from build123d import *

# Parameters (mm, degrees)
SKETCH2_R           = 2
BOSS_EXTRUDE1_DEPTH = 2.5
FILLET1_R           = 4
FILLET2_R           = 2


with BuildPart() as part:
    # Sketch2 → Boss-Extrude1 (new body)
    with BuildSketch(Plane.XY.offset(38.1)):
        Polygon((-27.5, 0), (27.5, 0), (27.5, 59.920564885), (-7.5, 59.920564885), (-7.5, 47.920564885), (15.5, 47.920564885), (15.5, 25.623759218), (1.876240782, 12), (-15.5, 12), (-15.5, 24), (-27.5, 24), (-27.5, 12), align=None)
        with Locations((-3.5, 56.920564885)):
            Circle(SKETCH2_R, mode=Mode.SUBTRACT)
        with Locations((-3.5, 50.920564885)):
            Circle(SKETCH2_R, mode=Mode.SUBTRACT)
        with Locations((4.5, 50.920564885)):
            Circle(SKETCH2_R, mode=Mode.SUBTRACT)
        with Locations((12.5, 50.920564885)):
            Circle(SKETCH2_R, mode=Mode.SUBTRACT)
        with Locations((4.5, 56.920564885)):
            Circle(SKETCH2_R, mode=Mode.SUBTRACT)
        with Locations((12.5, 56.920564885)):
            Circle(SKETCH2_R, mode=Mode.SUBTRACT)
        with Locations((20.5, 56.920564885)):
            Circle(SKETCH2_R, mode=Mode.SUBTRACT)
        Polygon((23.5, 4), (23.5, 47.920564885), (19.5, 47.920564885), (19.5, 23.966904969), (3.533095031, 8), (-19.190748402, 8), (-19.190748402, 20), (-23.5, 20), (-23.5, 8), (-23.5, 4), align=None, mode=Mode.SUBTRACT)
    extrude(amount=BOSS_EXTRUDE1_DEPTH)

    # Fillet1
    fillet1_edges = [part.edges().sort_by_distance(p)[0] for p in [
        (15.5, 25.623759218, 39.35),
        (15.5, 47.920564885, 39.35),
        (27.5, 0, 39.35),
        (-27.5, 0, 39.35),
        (-27.5, 24, 39.35),
        (-15.5, 24, 39.35),
        (-15.5, 12, 39.35),
        (1.876240782, 12, 39.35),
        (23.5, 4, 39.35),
        (19.5, 23.966904969, 39.35),
        (3.533095031, 8, 39.35),
    ]]
    fillet(fillet1_edges, radius=FILLET1_R)

    # Fillet2
    fillet2_edges = [part.edges().sort_by_distance(p)[0] for p in [
        (-7.5, 47.920564885, 39.35),
        (-7.5, 59.920564885, 39.35),
        (27.5, 59.920564885, 39.35),
        (-23.5, 4, 39.35),
        (23.5, 47.920564885, 39.35),
        (19.5, 47.920564885, 39.35),
        (-19.190748402, 8, 39.35),
        (-19.190748402, 20, 39.35),
        (-23.5, 20, 39.35),
    ]]
    fillet(fillet2_edges, radius=FILLET2_R - 0.0001)  # a hair under: the kernel refuses the full size


solid = part.part
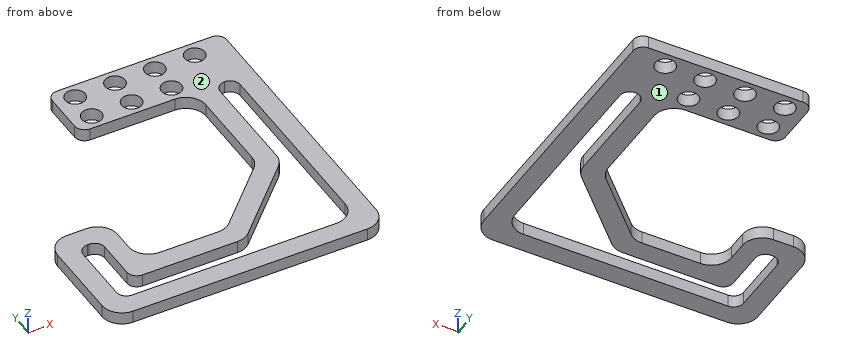
Can you work these out from the model? Positions are in its coordinate system, mm. Face numbers are marked on the shaded views. Give positions to 0.01 mm unless a question says otherwise; leave off trailing zeros. Loops run counter-clockwise (first coordinate to the right, second up) from the corner with the lowest first, then second, coordinate; pieces in that order, holes last. Notation, with made-up numbers: (74.5, 1.25) -> (117.5, 1.25) arc R21 cw to (117.5, 20.25) -> close; hole circle Ø8 at (57, -26). An arc over 180 degrees is marked (long way). Use one line per item in the form item = value.
1) If we section it at C-C (y = 52): Please give me the cut outline in (x, z), plus the area to 3 significant figures.
Answers:
outline = (-7.5, 38.1) -> (-5.18, 38.1) -> (-5.18, 40.6) -> (-7.5, 40.6) -> close; (-1.82, 38.1) -> (2.82, 38.1) -> (2.82, 40.6) -> (-1.82, 40.6) -> close; (6.18, 38.1) -> (10.82, 38.1) -> (10.82, 40.6) -> (6.18, 40.6) -> close; (14.18, 38.1) -> (27.5, 38.1) -> (27.5, 40.6) -> (14.18, 40.6) -> close
area = 62.2 mm²
2) If we section it at B-B (y = 40): Please give me the cut outline in (x, z), plus the area to 3 significant figures.
Answers:
outline = (15.5, 38.1) -> (19.5, 38.1) -> (19.5, 40.6) -> (15.5, 40.6) -> close; (23.5, 38.1) -> (27.5, 38.1) -> (27.5, 40.6) -> (23.5, 40.6) -> close
area = 20.0 mm²
3) Will these pins go through, and if not, where does the flat tip stop? pin 1 (1.2 mm diameter, centred on y = 52, z = 39, fed in from -X); pin 2 (1.2 mm diameter, centred on x = -21, z = 39.5, fed in from +Y); pin 3 (1.5 mm diameter, centred on x = -6.5, z = 39.5, fed in from +Y).
Answers:
pin_1 = -7.5
pin_2 = 24
pin_3 = 59.9
4) I need wall thicknesses on line 1 along Y through (x, z) = (-3.5, 39); line 2 along X through (y, z) = (39, 40.35); line 3 along Y through (x, z) = (20.5, 39.35). Which ranges of each line are inside material? Lowest first, please.
Answers:
line_1 = 0 to 4, 8 to 12, 47.92 to 48.92, 52.92 to 54.92, 58.92 to 59.92
line_2 = 15.5 to 19.5, 23.5 to 27.5
line_3 = 0 to 4.13, 47.65 to 54.92, 58.92 to 59.92
5) We'd pull the mould along Z, two halves only. Please class the marked faces 1 and 2: released by +Z, released by -Z, zero draft, split by the parting line, or undercut.
Answers:
face_1 = released by -Z
face_2 = released by +Z
6) If we section it at A-A (x = -3.5): Please give me the cut outline in (y, z), plus the area to 3 significant figures.
Answers:
outline = (0, 38.1) -> (4, 38.1) -> (4, 40.6) -> (0, 40.6) -> close; (8, 38.1) -> (12, 38.1) -> (12, 40.6) -> (8, 40.6) -> close; (47.92, 38.1) -> (48.92, 38.1) -> (48.92, 40.6) -> (47.92, 40.6) -> close; (52.92, 38.1) -> (54.92, 38.1) -> (54.92, 40.6) -> (52.92, 40.6) -> close; (58.92, 38.1) -> (59.92, 38.1) -> (59.92, 40.6) -> (58.92, 40.6) -> close
area = 30.0 mm²
7) If we section it at D-D (x = 20.5): Please give me the cut outline in (y, z).
Answers:
outline = (0, 38.1) -> (4.13, 38.1) -> (4.13, 40.6) -> (0, 40.6) -> close; (47.65, 38.1) -> (54.92, 38.1) -> (54.92, 40.6) -> (47.65, 40.6) -> close; (58.92, 38.1) -> (59.92, 38.1) -> (59.92, 40.6) -> (58.92, 40.6) -> close
